from build123d import *

# Parameters (mm, degrees)
F0_W     = 69.85
F0_H     = 69.85
F0_R     = 2
F3_DEPTH = 12.7
F1_R     = 31.353125
F4_DEPTH = 6.35
F2_R     = 11.1125
F5_DEPTH = 6.35


with BuildPart() as f3:
    # F0 (on Front) → F3 (new body)
    with BuildSketch(Plane.XZ):
        Rectangle(F0_W, F0_H)
        with Locations((-30.925, -30.925)):
            Circle(F0_R, mode=Mode.SUBTRACT)
        with Locations((30.925, -30.925)):
            Circle(F0_R, mode=Mode.SUBTRACT)
        with Locations((-30.925, 30.925)):
            Circle(F0_R, mode=Mode.SUBTRACT)
        with Locations((30.925, 30.925)):
            Circle(F0_R, mode=Mode.SUBTRACT)
    extrude(amount=F3_DEPTH)

    # F1 (on Front) → F4 (cut)
    with BuildSketch(Plane.XZ):
        Circle(F1_R)
    extrude(amount=F4_DEPTH, mode=Mode.SUBTRACT)

    # F2 (on Front) → F5 (join)
    with BuildSketch(Plane.XZ):
        Circle(F2_R)
    extrude(amount=F5_DEPTH)


solid = f3.part
The listing builds one solid part. Answer for the finished solid, in the listing's coordinates (mm). A direction names the side the tool comes from. Round coordinates to 2 decimals unless told otherwise and drop trailing zeros. Loops run counter-clockwise (first coordinate to the right, second up) from the corner with the lowest first, then second, coordinate; pieces in that order, holes last. Notation, with made-up numbers: M 66,12.25 L 112,12.25 A22 cw 112,51.25 Z; hole C 25.25,-12.75 d11. An arc over 180 degrees is marked long. Return JSON: item names as keys, results as strings.
Q1. Find section D-D, the plane x = 22.5. Determine the outline of the cut face in (y, z) (3 decimals), plus the area to 3 significant figures.
Results list:
{"outline": "M -12.7,-34.925 L 0,-34.925 L 0,-21.835 L -6.35,-21.835 L -6.35,21.835 L 0,21.835 L 0,34.925 L -12.7,34.925 Z", "area": "610 mm2"}
Q2. Find the intervals of material crossed by line 1 along Z through (x, y) = (0, -2.75) (1 decimal); line 2 along Z through (x, y) = (-31.5, -6.5) (3 decimals); line 3 along X through (y, z) = (-0.75, -2.5) (3 decimals), in increasing order. Write a range as from..to.
Results list:
{"line 1": "z = -34.9..-31.4, -11.1..11.1, 31.4..34.9", "line 2": "z = -34.925..-32.841, -29.009..29.009, 32.841..34.925", "line 3": "x = -34.925..-31.253, -10.828..10.828, 31.253..34.925"}
Q3. The mould has two halves that part along X. Classify faces 3 (the face through (0, -12.7, 0)), 4 (the face through (-34.925, -6, 0)), 5 (the face through (13, -6.35, 0)), 6 (the face through (-29.02, -6.26, -30.32)): released by +X, released by -X, zero draft, split by the parting line, or undercut.
Results list:
{"face 3": "zero draft", "face 4": "released by -X", "face 5": "undercut", "face 6": "undercut"}
Q4. Which of the six approach directions +Z, -Z, +X, -X, +Y, -Y give full straight-line access (tool end or side, diameter ignored) to faces 1 (the face through (0, -6, -34.925)), 2 (the face through (-24.88, -3.13, -19.08))?
Results list:
{"face 1": "-Z, +X, -X, +Y, -Y", "face 2": "+Y"}
Q5. Each of these flat-tipped pins is pushed along its axis until it touches: pin 1 Ø4 at (x, z) = (-3.5, 11.5) entering from +Y; pin 2 Ø6 at (x, z) = (20, 13.5) entering from +Y. Where does it stop, or does it pass through?
Results list:
{"pin 1": "stops at y = 0", "pin 2": "stops at y = -6.35"}
Q6. Find section A-A, the plane y = -1. Determine the outline of the cut face in (x, z) (1 decimal), plus the area to 3 significant figures.
Results list:
{"outline": "M -34.9,-34.9 L 34.9,-34.9 L 34.9,34.9 L -34.9,34.9 Z; C 0,0 d22.2; hole C -30.9,-30.9 d4; hole C -30.9,30.9 d4; hole C 0,0 d62.7; hole C 30.9,-30.9 d4; hole C 30.9,30.9 d4", "area": "2,130 mm2"}
